```python
from build123d import *

# Parameters (mm, degrees)
SKETCH1_W           = 8.0264
SKETCH1_H           = 8.0264
BOSS_EXTRUDE1_DEPTH = 2.286
SKETCH2_R           = 4.091254354
BOSS_EXTRUDE2_DEPTH = 3.302
SKETCH3_R           = 1.040494651
CUT_EXTRUDE1_DEPTH  = 3.302
SKETCH8_W           = 6.096
SKETCH8_H           = 13.5255
BOSS_EXTRUDE6_DEPTH = 0.127
SKETCH9_W           = 8.0264
SKETCH9_H           = 8.0264
BOSS_EXTRUDE7_DEPTH = 0.254


with BuildPart() as part:
    # Sketch1 → Boss-Extrude1 (new body)
    with BuildSketch(Plane.XY):
        Rectangle(SKETCH1_W, SKETCH1_H)
    extrude(amount=BOSS_EXTRUDE1_DEPTH)

    # Sketch2 → Boss-Extrude2 (add)
    with BuildSketch(Plane.XY.offset(2.286)):
        with Locations(Location((0, 0, 0), (0, 0, 168.79012288))):
            Circle(SKETCH2_R)
    extrude(amount=BOSS_EXTRUDE2_DEPTH)

    # Sketch3 → Cut-Extrude1 (cut)
    with BuildSketch(Plane.XY.offset(5.588)):
        Circle(SKETCH3_R)
    extrude(amount=-CUT_EXTRUDE1_DEPTH, mode=Mode.SUBTRACT)

    # Sketch8 → Boss-Extrude6 (add)
    with BuildSketch(Plane(origin=(0, 0, 0), x_dir=(-1, 0, 0), z_dir=(0, 0, -1))):
        with Locations((0, -3.71475)):
            Rectangle(SKETCH8_W, SKETCH8_H)
    extrude(amount=BOSS_EXTRUDE6_DEPTH)

    # Sketch9 → Boss-Extrude7 (add)
    with BuildSketch(Plane(origin=(0, 0, 0), x_dir=(-1, 0, 0), z_dir=(0, 0, -1))):
        Rectangle(SKETCH9_W, SKETCH9_H)
    extrude(amount=BOSS_EXTRUDE7_DEPTH)


solid = part.part
```
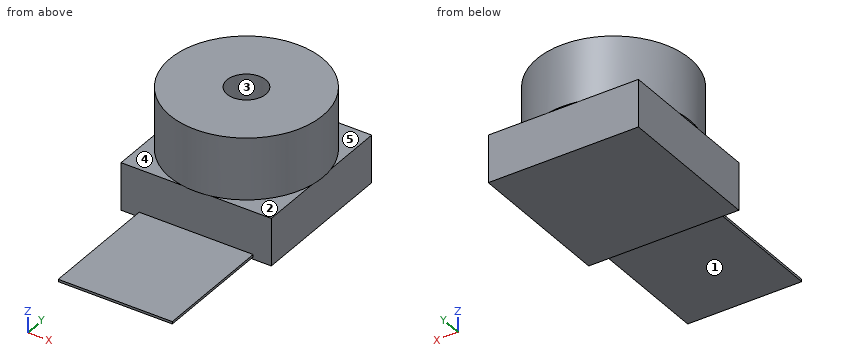
CAD build for the part. Positions are in the model's coordinates, mm. Face numbers are marked on the shaded views. A direction names the side the tool comes from. Give positions to 0.01 mm unless a question says otherwise; leave off trailing zeros. Write each loop counter-clockwise with the first axis right and the second up, starting at its lowest first coordinate (ties: lowest second). Pieces come first, ordered by that corner, then holes. Notation, with made-up numbers: (-33.75, -27) -> (-26.75, -27) arc R18 cw to (-26.75, 3) -> close; hole circle Ø4 at (-15, -27.75). An arc over 180 degrees is marked (long way). Write each question's results on one line, items separated by ' | '.
1. Cut at A-A, the plane y = 0. Write the cut outline in (x, z), then the cut area to 3 significant figures.
Geometry check:
outline: (-4.09, 2.29) -> (-4.01, 2.29) -> (-4.01, -0.25) -> (4.01, -0.25) -> (4.01, 2.29) -> (4.09, 2.29) -> (4.09, 5.59) -> (1.04, 5.59) -> (1.04, 2.29) -> (-1.04, 2.29) -> (-1.04, 5.59) -> (-4.09, 5.59) -> close | area: 40.5 mm²
2. Cut at C-C, the plane z = 3.6. Write the cut outline in (x, y), then the cut area to 3 significant figures.
Geometry check:
outline: circle Ø8.18 at (0, 0); hole circle Ø2.08 at (0, 0) | area: 49.2 mm²
3. Wall check: probe 1 along Y at (x, z) = (0, 4.95); probe 2 along Y at (x, z) = (2.75, 0.95); probe 3 along Z at (x, y) = (0, 0.25). Give the ranges that are in metal, low to high. Write a range as [from, to].
Geometry check:
probe 1: [-4.09, -1.04], [1.04, 4.09] | probe 2: [-4.01, 4.01] | probe 3: [-0.25, 2.29]
4. Cut at D-D, the plane z = 1. Write the cut outline in (x, y).
Geometry check:
outline: (-4.01, -4.01) -> (4.01, -4.01) -> (4.01, 4.01) -> (-4.01, 4.01) -> close
5. Cut at B-B, the plane x = 0. Write the cut outline in (y, z), then the cut area to 3 significant figures.
Geometry check:
outline: (-10.48, -0.13) -> (-4.01, -0.13) -> (-4.01, -0.25) -> (4.01, -0.25) -> (4.01, 2.29) -> (4.09, 2.29) -> (4.09, 5.59) -> (1.04, 5.59) -> (1.04, 2.29) -> (-1.04, 2.29) -> (-1.04, 5.59) -> (-4.09, 5.59) -> (-4.09, 2.29) -> (-4.01, 2.29) -> (-4.01, 0) -> (-10.48, 0) -> close | area: 41.4 mm²
6. Drop flat-ended pins along their axis: P1, Ø1.8, axis at x = -1.5, y = -6.5, coming from the +Z side; P2, Ø3, axis at x = -2.5, z = 1, coming from the +Y side; P3, Ø1.7, axis at x = 0, y = 0, coming from the +Z side. Give the stop position or say it passes through.
Geometry check:
P1: z = 0 | P2: y = 4.01 | P3: z = 2.29
7. Which spindle directions (+Z, -Z, +X, -X, +Y, -Y) get a long thin tool onto all of the face, cutting with end or side? Do the marked faces 1, 2, 3, 4 and 5. Say none if no direction does.
Geometry check:
face 1: -Z, +X, -X, -Y | face 2: +Z, +X, -Y | face 3: +Z | face 4: +Z, -X, -Y | face 5: +Z, +X, +Y
